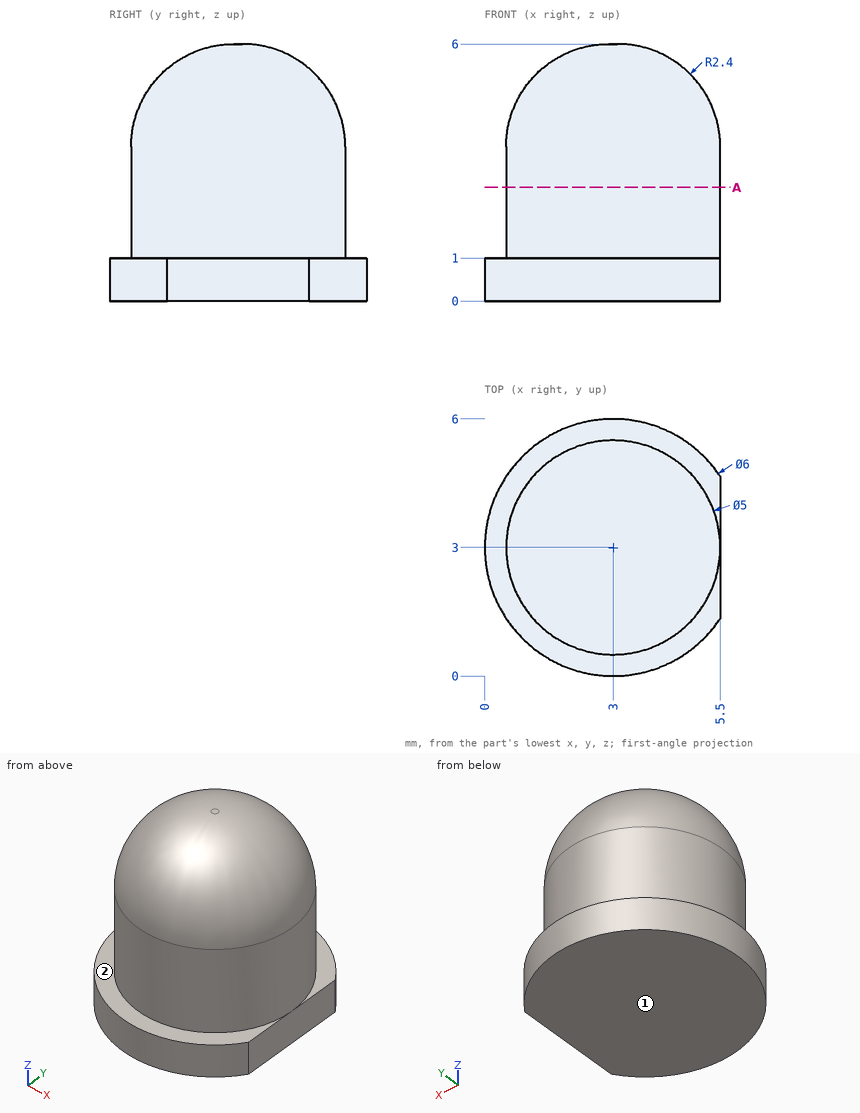
Input: dimensioned drawing with shaded views. Units: mm. Origin: part minimum x, y, z. A direction names the side the tool comes from. Round coordinates to 2 decimals unless told otherwise and drop trailing zeros. Write each loop counter-clockwise with the first axis right and the second up, starting at its lowest first coordinate (ties: lowest second). Pieces come first, ordered by that corner, then holes. Notation, with made-up numbers: (22.25, -1.5) -> (63.25, -1.5) arc R17 cw to (63.25, 14.5) -> close; hole circle Ø7 at (-0.5, 63). An arc over 180 degrees is marked (long way). Use CSV: the item, a comma, the result in double quotes. Start each with the question number.
Q1. First-contact query: pin 1 Ø1 at (x, y) = (4.5, 3) entering from +Z; pin 2 Ø3 at (x, y) = (2, 2.5) entering from +Z; pin 3 Ø2 at (x, y) = (4.5, 5) entering from +Z. Flat tips, straight axial feed; report the tip coordinate or a pass-through.
Q2. Reachability of the marked faces 1 and 2 from +Z, -Z, +X, -X, +Y, -Y: full face, straight path, thin tool, end or side. Return the list, or none.
Q3. Line query: L1, parallel to Z at x = 1.95, y = 5.4; L2, parallel to X at y = 3.1, z = 1.85; L3, parallel to Y at x = 4.95, z = 3.05. Output: solid intervals per line, ascending.
Q4. Section A-A (z = 2.65). Return loops of the section in (x, y), plus the area to 3 significant figures.
Result sheet:
1,pin 1,"z = 5.82"
1,pin 2,"z = 6"
1,pin 3,"z = 5.55"
2,face 1,"-Z, +X, -X, +Y, -Y"
2,face 2,"+Z"
3,L1,"0 to 1"
3,L2,"0.5 to 5.5"
3,L3,"1.44 to 4.56"
4,outline,"circle Ø5 at (3, 3)"
4,area,"19.6 mm²"
